from build123d import *

# Parameters (mm, degrees)
F0_R     = 9.5
F1_DEPTH = 14
F2_W     = 5.25
F2_H     = 5.25
F3_DEPTH = 10


with BuildPart() as f1:
    # F0 (on Front) → F1 (new body)
    with BuildSketch(Plane.XZ):
        Circle(F0_R)
    extrude(amount=F1_DEPTH)

    # F2 (on face) → F3 (cut)
    with BuildSketch(Plane(origin=(0, 0, 0), x_dir=(-1, 0, 0), z_dir=(0, 1, 0))):
        Rectangle(F2_W, F2_H)
    extrude(amount=-F3_DEPTH, mode=Mode.SUBTRACT)


solid = f1.part
The model under review builds one solid part; all positions refer to its coordinate system, in mm. A direction names the side the tool comes from. Round coordinates to 2 decimals unless told otherwise and drop trailing zeros. Loops run counter-clockwise (first coordinate to the right, second up) from the corner with the lowest first, then second, coordinate; pieces in that order, holes last. Notation, with made-up numbers: (38.25, -16) -> (89.25, -16) arc R28 ccw to (89.25, 20) -> close; hole circle Ø4 at (-39, 74). An arc over 180 degrees is marked (long way). Write item = value, one per line. Start each with the question number.
Item 1: Take a section at B-B on x = 0. Give the boundary of the cut face in (y, z) (3 decimals).
Item 2: Take a section at A-A on y = -1.75. Give the boundary of the cut face in (x, z) (3 decimals).
Item 3: Take a section at D-D on y = -11.75. Give the boundary of the cut face in (x, z), plus the area to 3 significant figures.
Item 4: To check wall thickness, follow L1, parallel to Z at x = -0.25, y = -1.75 (3 decimals); L2, parallel to X at y = -6.5, z = -1 (3 decimals); L3, parallel to Z at x = -2, y = -6 (3 decimals). State the ranges of each line that lie inside material, in increasing order.
Item 5: For faces 5 (the flat face through (4, 0, 0)), 6 (the flat face through (2.625, -5, 0)), list the 3-axis set-ups (+Z, -Z, +X, -X, +Y, -Y) from which the entire face can be reached by the end or side of a thin tool; tool diameter is ignored.
Item 6: Insertion check: pin 1 (1.6 mm diameter, centred on x = 0, z = 1, fed in from +Y); pin 2 (5 mm diameter, centred on x = 7.5, y = -3.5, fed in from -Z); pin 3 (4 mm diameter, centred on y = -1.5, z = 7.5, fed in from -X). Each pin has a flat end and moves straight along its axis. Give the tip position at first contact, or say it passes through.
Item 7: Take a section at C-C on z = 0. Give the boundary of the cut face in (x, y) (3 decimals).
Item 8: Mouldability with a two-part tool opening along X and no side actions: class faces 1 (the flat face through (0, -14, 0)), 2 (the flat face through (-2.625, -5, 0)), 3 (the cylindrical face through (4.38, -6.9, -8.43)), 4 (the flat face through (0, -10, 0)) as released by +X, released by -X, zero draft, split by the parting line, or undercut.
Result:
q1.outline = (-14, -9.5) -> (0, -9.5) -> (0, -2.625) -> (-10, -2.625) -> (-10, 2.625) -> (0, 2.625) -> (0, 9.5) -> (-14, 9.5) -> close
q2.outline = circle Ø19 at (0, 0); hole (-2.625, -2.625) -> (2.625, -2.625) -> (2.625, 2.625) -> (-2.625, 2.625) -> close
q3.outline = circle Ø19 at (0, 0)
q3.area = 284 mm²
q4.L1 = -9.497 to -2.625, 2.625 to 9.497
q4.L2 = -9.447 to -2.625, 2.625 to 9.447
q4.L3 = -9.287 to -2.625, 2.625 to 9.287
q5.face_5 = +Z, -Z, +X, -X, +Y
q5.face_6 = +Y
q6.pin_1 = -10
q6.pin_2 = -8.08
q6.pin_3 = -7.75
q7.outline = (-9.5, -14) -> (9.5, -14) -> (9.5, 0) -> (2.625, 0) -> (2.625, -10) -> (-2.625, -10) -> (-2.625, 0) -> (-9.5, 0) -> close
q8.face_1 = zero draft
q8.face_2 = undercut
q8.face_3 = split by the parting line
q8.face_4 = undercut
